Verification items for the finished model (mm, model axes). Face numbers are marked on the shaded views. Coordinates: 2 decimals unless noted, no trailing zeros. Order: outer loops, then holes, each group sorted by start corner. A loop starts at its lowest first (then second) coordinate and runs counter-clockwise, first axis right, second up. Notation, with made-up numbers: M 65,86 L 106,86 A23 ccw 106,94 Z; hole C -15,-9 d4. An arc over 180 degrees is marked long. Return JSON: item names as keys, results as strings.
```python
from build123d import *

# Parameters (mm, degrees)
SKETCH1_R           = 22.479
BOSS_EXTRUDE1_DEPTH = 6.35
SKETCH2_R           = 25.4
BOSS_EXTRUDE2_DEPTH = 3.81
SKETCH3_R           = 8.9916
CUT_EXTRUDE1_DEPTH  = 3.81
SKETCH4_R           = 3.175
CUT_EXTRUDE2_DEPTH  = 37.477972806


with BuildPart() as part:
    # Sketch1 → Boss-Extrude1 (new body)
    with BuildSketch(Plane(origin=(0, 0, 0), x_dir=(1, 0, 0), z_dir=(0, 1, 0))):
        with Locations(Location((0, 0, 0), (0, 0, 270))):
            Circle(SKETCH1_R)
    extrude(amount=BOSS_EXTRUDE1_DEPTH)

    # Sketch2 → Boss-Extrude2 (add)
    with BuildSketch(Plane(origin=(0, 6.35, 0), x_dir=(1, 0, 0), z_dir=(0, 1, 0))):
        with Locations(Location((0, 0, 0), (0, 0, 90))):
            Circle(SKETCH2_R)
    extrude(amount=BOSS_EXTRUDE2_DEPTH)

    # Sketch3 → Cut-Extrude1 (cut)
    with BuildSketch(Plane.XZ):
        with Locations(Location((0, 0, 0), (0, 0, 270))):
            Circle(SKETCH3_R)
    extrude(amount=-CUT_EXTRUDE1_DEPTH, mode=Mode.SUBTRACT)

    # Sketch4 → Cut-Extrude2 (cut, through all)
    with BuildSketch(Plane.XZ.offset(-3.81)):
        with Locations(Location((0, 0, 0), (0, 0, 270))):
            Circle(SKETCH4_R)
    extrude(amount=-CUT_EXTRUDE2_DEPTH, mode=Mode.SUBTRACT)


solid = part.part
```
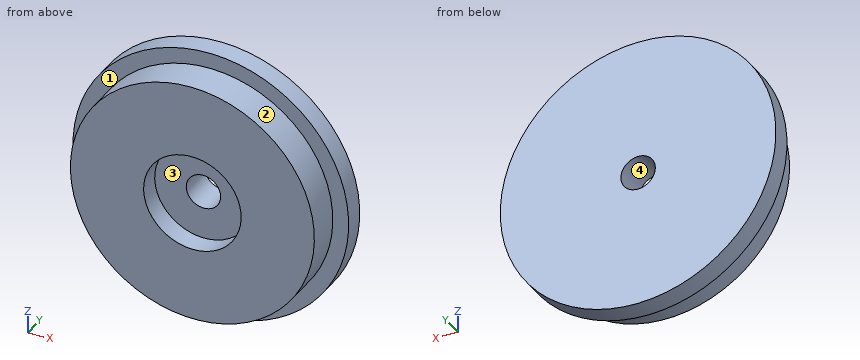
Q1. Cross-section at D-D, the plane x = -19.5. Record the boundary of the cut face in (y, z), and give its area (3 significant figures).
Values:
{"outline": "M 0,-11.18 L 6.35,-11.18 L 6.35,-16.28 L 10.16,-16.28 L 10.16,16.28 L 6.35,16.28 L 6.35,11.18 L 0,11.18 Z", "area": "266 mm^2"}
Q2. Go/stop test with flat-tipped pins: pin 1 (5.5 mm diameter, centred on x = -3, z = -4, fed in from -Y); pin 2 (2 mm diameter, centred on y = 4.5, z = 13.5, fed in from -X). Record where each tip stops, or that it passes through.
Values:
{"pin 1": "y = 3.81", "pin 2": "x = -18.68"}
Q3. Material ranges on line 1 along X through (y, z) = (8.25, 0) (3 decimals); line 2 along X through (y, z) = (5.25, 0) (3 decimals); line 3 along Y through (x, z) = (-9, 22), recorded low to high.
Values:
{"line 1": "-25.4 to -3.175, 3.175 to 25.4", "line 2": "-22.479 to -3.175, 3.175 to 22.479", "line 3": "6.35 to 10.16"}
Q4. Cross-section at B-B, the plane z = 0. Record the boundary of the cut face in (x, y) (3 decimals).
Values:
{"outline": "M -25.4,6.35 L -22.479,6.35 L -22.479,0 L -8.992,0 L -8.992,3.81 L -3.175,3.81 L -3.175,10.16 L -25.4,10.16 Z; M 3.175,3.81 L 8.992,3.81 L 8.992,0 L 22.479,0 L 22.479,6.35 L 25.4,6.35 L 25.4,10.16 L 3.175,10.16 Z"}
Q5. Draft check along Z on the marked faces 1, 2, 3 and 4. Enter one of: pulls with the +Z half, pulls with the -Z half, needs draft (parallel to the pull), parting line crosses it, or undercut.
Values:
{"face 1": "needs draft", "face 2": "parting line crosses it", "face 3": "undercut", "face 4": "undercut"}
Q6. Cross-section at C-C, the plane y = 4.75. Record the boundary of the cut face in (x, z) (3 decimals).
Values:
{"outline": "C 0,0 d44.958; hole C 0,0 d6.35"}
Q7. Cross-section at A-A, the plane x = 0. Record the boundary of the cut face in (y, z) (3 decimals).
Values:
{"outline": "M 0,-22.479 L 6.35,-22.479 L 6.35,-25.4 L 10.16,-25.4 L 10.16,-3.175 L 3.81,-3.175 L 3.81,-8.992 L 0,-8.992 Z; M 0,8.992 L 3.81,8.992 L 3.81,3.175 L 10.16,3.175 L 10.16,25.4 L 6.35,25.4 L 6.35,22.479 L 0,22.479 Z"}
